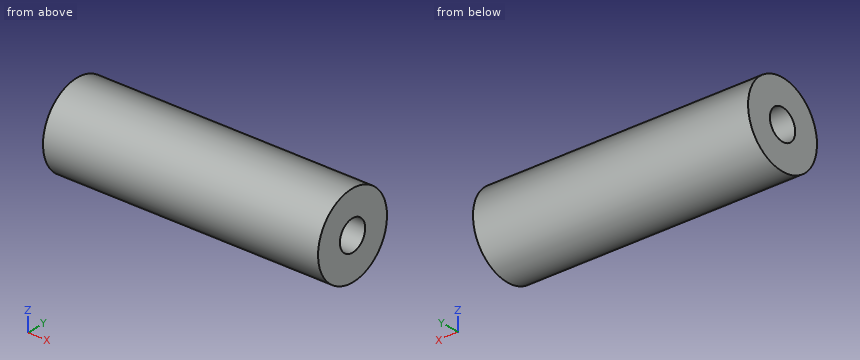
```python
from build123d import *

# Parameters (mm, degrees)
OBJ1_R     = 1.1
OBJ1_DEPTH = 20
OBJ2     = 3
OBJ3 = 20


with BuildPart() as obj1:
    # obj1 → obj1 (new body)
    with BuildSketch(Plane(origin=(34.9, -1, 43), x_dir=(0, 0, -1), z_dir=(1, 0, 0))):
        Circle(OBJ1_R)
    extrude(amount=OBJ1_DEPTH)


with BuildPart() as hinge_left:
    with BuildSketch(Plane(origin=(34.9, -1, 43), x_dir=(0, 0, -1), z_dir=(1, 0, 0))):
        Circle(OBJ2)
    extrude(amount=OBJ3)

    # hinge_left: cut obj1
    add(obj1.part, mode=Mode.SUBTRACT)


solid = hinge_left.part
```
Can you work these out from the model? Positions are in its coordinate system, mm. Coordinates: 2 decimals unless noted, no trailing zeros. Loops run counter-clockwise (first coordinate to the right, second up) from the corner with the lowest first, then second, coordinate; pieces in that order, holes last.
Item 1: I'm going to push flat-ended pins straight in: pin 1 (2 mm diameter, centred on x = 39, z = 44.5, fed in from -Y); pin 2 (1.5 mm diameter, centred on x = 40, y = 0.5, fed in from +Z); pin 3 (2 mm diameter, centred on x = 52.5, z = 41, fed in from -Y). Where does each tip first touch, or does it pass through?
Answers below:
pin 1: stops at y = -3.96
pin 2: stops at z = 45.9
pin 3: stops at y = -3.83
Item 2: Suppose I cut it at C-C (x = 45.75). Please give me the cut outline in (y, z).
Answers below:
outline: circle Ø6 at (-1, 43); hole circle Ø2.2 at (-1, 43)
Item 3: Suppose I cut it at B-B (z = 43). Please give me the cut outline in (x, y).
Answers below:
outline: (34.9, -4) - (54.9, -4) - (54.9, -2.1) - (34.9, -2.1) - close; (34.9, 0.1) - (54.9, 0.1) - (54.9, 2) - (34.9, 2) - close
Item 4: Suppose I cut it at A-A (y = -1). Please give me the cut outline in (x, z), then the cut area to 3 significant figures.
Answers below:
outline: (34.9, 40) - (54.9, 40) - (54.9, 41.9) - (34.9, 41.9) - close; (34.9, 44.1) - (54.9, 44.1) - (54.9, 46) - (34.9, 46) - close
area: 76.0 mm2
Item 5: Suppose I cut it at D-D (z = 41.2). Please give me the cut outline in (x, y), then the cut area to 3 significant figures.
Answers below:
outline: (34.9, -3.4) - (54.9, -3.4) - (54.9, 1.4) - (34.9, 1.4) - close
area: 96.0 mm2
Item 6: Please list where these lines run through material, in increasing order: L1, parallel to Y at x = 39, z = 43; L2, parallel to Z at x = 49.75, y = -1.4; L3, parallel to Z at x = 52, y = -0.4.
Answers below:
L1: y = -4 to -2.1, 0.1 to 2
L2: z = 40.03 to 41.98, 44.02 to 45.97
L3: z = 40.06 to 42.08, 43.92 to 45.94
